Source: CAD feature listing. Evaluate the final solid. Frame: model axes, mm. Give positions to 0.01 mm unless a question says otherwise; leave off trailing zeros. Order: outer loops, then holes, each group sorted by start corner. A loop starts at its lowest first (then second) coordinate and runs counter-clockwise, first axis right, second up.
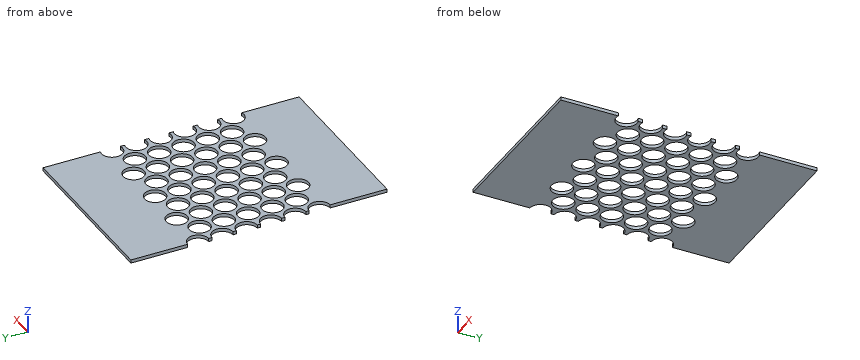
from build123d import *

# Parameters (mm, degrees)
SKETCH061_W     = 445
SKETCH061_H     = 232
PAD023_DEPTH    = 3
SKETCH062_R     = 9.5
POCKET038_DEPTH = 5
FILLET008_R     = 2
SKETCH063_R     = 7
POCKET039_DEPTH = 10.001
POCKET052_DEPTH = 5


with BuildPart() as part:
    # Sketch061 → Pad023 (new body)
    with BuildSketch(Plane.XY):
        Rectangle(SKETCH061_W, SKETCH061_H)
    extrude(amount=PAD023_DEPTH)

    # Sketch062 (on Face6 of Pad023) → Pocket038 (cut)
    with BuildSketch(Plane.XY.offset(3)):
        with Locations((-171, 55)):
            Circle(SKETCH062_R)
        with Locations((-171, 33)):
            Circle(SKETCH062_R)
        with Locations((-171, 11)):
            Circle(SKETCH062_R)
        with Locations((-171, -11)):
            Circle(SKETCH062_R)
        with Locations((-171, -33)):
            Circle(SKETCH062_R)
        with Locations((-171, -55)):
            Circle(SKETCH062_R)
        with Locations((-152, 44)):
            Circle(SKETCH062_R)
        with Locations((-152, 22)):
            Circle(SKETCH062_R)
        with Locations((-152, 0)):
            Circle(SKETCH062_R)
        with Locations((-152, -22)):
            Circle(SKETCH062_R)
        with Locations((-152, -44)):
            Circle(SKETCH062_R)
        with Locations((-133, 55)):
            Circle(SKETCH062_R)
        with Locations((-133, 33)):
            Circle(SKETCH062_R)
        with Locations((-133, 11)):
            Circle(SKETCH062_R)
        with Locations((-133, -11)):
            Circle(SKETCH062_R)
        with Locations((-133, -33)):
            Circle(SKETCH062_R)
        with Locations((-133, -55)):
            Circle(SKETCH062_R)
        with Locations((-114, 44)):
            Circle(SKETCH062_R)
        with Locations((-114, 22)):
            Circle(SKETCH062_R)
        with Locations((-114, 0)):
            Circle(SKETCH062_R)
        with Locations((-114, -22)):
            Circle(SKETCH062_R)
        with Locations((-114, -44)):
            Circle(SKETCH062_R)
        with Locations((-95, 55)):
            Circle(SKETCH062_R)
        with Locations((-95, 33)):
            Circle(SKETCH062_R)
        with Locations((-95, 11)):
            Circle(SKETCH062_R)
        with Locations((-95, -11)):
            Circle(SKETCH062_R)
        with Locations((-95, -33)):
            Circle(SKETCH062_R)
        with Locations((-95, -55)):
            Circle(SKETCH062_R)
        with Locations((-76, -44)):
            Circle(SKETCH062_R)
        with Locations((-76, -22)):
            Circle(SKETCH062_R)
        with Locations((-76, 0)):
            Circle(SKETCH062_R)
        with Locations((-76, 22)):
            Circle(SKETCH062_R)
        with Locations((-76, 44)):
            Circle(SKETCH062_R)
        with Locations((-57, 55)):
            Circle(SKETCH062_R)
        with Locations((-57, 33)):
            Circle(SKETCH062_R)
        with Locations((-57, 11)):
            Circle(SKETCH062_R)
        with Locations((-57, -11)):
            Circle(SKETCH062_R)
        with Locations((-57, -33)):
            Circle(SKETCH062_R)
        with Locations((-38, 44)):
            Circle(SKETCH062_R)
        with Locations((-38, 22)):
            Circle(SKETCH062_R)
        with Locations((-38, 0)):
            Circle(SKETCH062_R)
        with Locations((-38, -22)):
            Circle(SKETCH062_R)
        with Locations((-38, -44)):
            Circle(SKETCH062_R)
        with Locations((-57, -55)):
            Circle(SKETCH062_R)
        with Locations((-19, 55)):
            Circle(SKETCH062_R)
        with Locations((-19, 33)):
            Circle(SKETCH062_R)
        with Locations((-19, 11)):
            Circle(SKETCH062_R)
        with Locations((-19, -11)):
            Circle(SKETCH062_R)
        with Locations((-19, -33)):
            Circle(SKETCH062_R)
        with Locations((-19, -55)):
            Circle(SKETCH062_R)
        with Locations((0, -44)):
            Circle(SKETCH062_R)
        with Locations((0, -22)):
            Circle(SKETCH062_R)
        Circle(SKETCH062_R)
        with Locations((0, 22)):
            Circle(SKETCH062_R)
        with Locations((0, 44)):
            Circle(SKETCH062_R)
        with Locations((19, 55)):
            Circle(SKETCH062_R)
        with Locations((19, 33)):
            Circle(SKETCH062_R)
        with Locations((19, 11)):
            Circle(SKETCH062_R)
        with Locations((19, -11)):
            Circle(SKETCH062_R)
        with Locations((19, -33)):
            Circle(SKETCH062_R)
        with Locations((19, -55)):
            Circle(SKETCH062_R)
        with Locations((38, -44)):
            Circle(SKETCH062_R)
        with Locations((38, -22)):
            Circle(SKETCH062_R)
        with Locations((38, 0)):
            Circle(SKETCH062_R)
        with Locations((38, 22)):
            Circle(SKETCH062_R)
        with Locations((38, 44)):
            Circle(SKETCH062_R)
        with Locations((57, 55)):
            Circle(SKETCH062_R)
        with Locations((57, 33)):
            Circle(SKETCH062_R)
        with Locations((57, 11)):
            Circle(SKETCH062_R)
        with Locations((57, -11)):
            Circle(SKETCH062_R)
        with Locations((76, 0)):
            Circle(SKETCH062_R)
        with Locations((76, 22)):
            Circle(SKETCH062_R)
        with Locations((76, 44)):
            Circle(SKETCH062_R)
        with Locations((57, -33)):
            Circle(SKETCH062_R)
        with Locations((57, -55)):
            Circle(SKETCH062_R)
        with Locations((76, -44)):
            Circle(SKETCH062_R)
        with Locations((76, -22)):
            Circle(SKETCH062_R)
        with Locations((95, 55)):
            Circle(SKETCH062_R)
        with Locations((95, 33)):
            Circle(SKETCH062_R)
        with Locations((95, 11)):
            Circle(SKETCH062_R)
        with Locations((95, -11)):
            Circle(SKETCH062_R)
        with Locations((95, -33)):
            Circle(SKETCH062_R)
        with Locations((95, -55)):
            Circle(SKETCH062_R)
        with Locations((114, 44)):
            Circle(SKETCH062_R)
        with Locations((114, 22)):
            Circle(SKETCH062_R)
        with Locations((114, 0)):
            Circle(SKETCH062_R)
        with Locations((114, -22)):
            Circle(SKETCH062_R)
        with Locations((114, -44)):
            Circle(SKETCH062_R)
        with Locations((133, 55)):
            Circle(SKETCH062_R)
        with Locations((133, 33)):
            Circle(SKETCH062_R)
        with Locations((133, 11)):
            Circle(SKETCH062_R)
        with Locations((133, -11)):
            Circle(SKETCH062_R)
        with Locations((133, -33)):
            Circle(SKETCH062_R)
        with Locations((133, -55)):
            Circle(SKETCH062_R)
        with Locations((152, 44)):
            Circle(SKETCH062_R)
        with Locations((152, 22)):
            Circle(SKETCH062_R)
        with Locations((152, 0)):
            Circle(SKETCH062_R)
        with Locations((152, -22)):
            Circle(SKETCH062_R)
        with Locations((152, -44)):
            Circle(SKETCH062_R)
        with Locations((171, 55)):
            Circle(SKETCH062_R)
        with Locations((171, 33)):
            Circle(SKETCH062_R)
        with Locations((171, 11)):
            Circle(SKETCH062_R)
        with Locations((171, -11)):
            Circle(SKETCH062_R)
        with Locations((171, -33)):
            Circle(SKETCH062_R)
        with Locations((171, -55)):
            Circle(SKETCH062_R)
    extrude(amount=-POCKET038_DEPTH, mode=Mode.SUBTRACT)

    # Fillet008
    fillet008_edges = [part.edges().sort_by_distance(p)[0] for p in [
        (-222.5, -116, 1.5),
        (222.5, -116, 1.5),
        (222.5, 116, 1.5),
        (-222.5, 116, 1.5),
    ]]
    fillet(fillet008_edges, radius=FILLET008_R)

    # Sketch063 → Pocket039 (cut, through all)
    with BuildSketch(Plane.XY.offset(10)):
        with Locations((197.939534, 0)):
            Circle(SKETCH063_R)
    extrude(amount=-POCKET039_DEPTH, mode=Mode.SUBTRACT)

    # Sketch080 (on Face5 of Pocket039) → Pocket052 (cut)
    with BuildSketch(Plane.XY.offset(3)):
        Polygon((-295.981628, 170.85997), (-95, 181.693848), (-95, -229.391144), (60, -229.391144), (60, 193.129593), (437.109833, 193.129593), (437.109833, -331.1091), (-295.981628, -331.1091), align=None)
    extrude(amount=-POCKET052_DEPTH, mode=Mode.SUBTRACT)


solid = part.part
(1) Section D-D, the plane x = -32.5. Return loops of the section in (y, z), plus the area to 3 significant figures.
(2) Pin query (flat end, axial travel): pin 1 Ø17 at (x, y) = (38, 22) entering from +Z. Return the tip coordinate at first contact, or that it passes through.
(3) Line query: line 1 along Y through (x, z) = (-76, 1.3); line 2 along Y through (x, z) = (40, 2.65). Output: solid intervals per line, ascending.
(4) Section A-A, the plane x = -57. Return loops of the section in (y, z).
(5) Section C-C, the plane y = 58.5. Return loops of the section in (x, z), plus the area to 3 significant figures.
(6) Section B-B, the plane y = 5. Count the separate pieces of the cut face and the enclosed holes in it, plus the area to 3 significant figures.
Checks:
1. outline: (-116, 0) - (-51.75, 0) - (-51.75, 3) - (-116, 3) - close; (-36.25, 0) - (-29.75, 0) - (-29.75, 3) - (-36.25, 3) - close; (-14.25, 0) - (-7.75, 0) - (-7.75, 3) - (-14.25, 3) - close; (7.75, 0) - (14.25, 0) - (14.25, 3) - (7.75, 3) - close; (29.75, 0) - (36.25, 0) - (36.25, 3) - (29.75, 3) - close; (51.75, 0) - (116, 0) - (116, 3) - (51.75, 3) - close
1. area: 464 mm2
2. pin 1: passes through
3. line 1: y = -116 to -53.5, -34.5 to -31.5, -12.5 to -9.5, 9.5 to 12.5, 31.5 to 34.5, 53.5 to 116
3. line 2: y = -116 to -53.29, -34.71 to -31.29, -12.71 to -9.29, 9.29 to 12.71, 31.29 to 34.71, 53.29 to 116
4. outline: (-116, 0) - (-64.5, 0) - (-64.5, 3) - (-116, 3) - close; (-45.5, 0) - (-42.5, 0) - (-42.5, 3) - (-45.5, 3) - close; (-23.5, 0) - (-20.5, 0) - (-20.5, 3) - (-23.5, 3) - close; (-1.5, 0) - (1.5, 0) - (1.5, 3) - (-1.5, 3) - close; (20.5, 0) - (23.5, 0) - (23.5, 3) - (20.5, 3) - close; (42.5, 0) - (45.5, 0) - (45.5, 3) - (42.5, 3) - close; (64.5, 0) - (116, 0) - (116, 3) - (64.5, 3) - close
5. outline: (-86.17, 0) - (-65.83, 0) - (-65.83, 3) - (-86.17, 3) - close; (-48.17, 0) - (-27.83, 0) - (-27.83, 3) - (-48.17, 3) - close; (-10.17, 0) - (10.17, 0) - (10.17, 3) - (-10.17, 3) - close; (27.83, 0) - (48.17, 0) - (48.17, 3) - (27.83, 3) - close
5. area: 244 mm2
6. separate pieces: 8
6. enclosed holes: 0
6. area: 85.4 mm2
